The listing builds one solid part. Answer for the finished solid, in the listing's coordinates (mm). A direction names the side the tool comes from. Round coordinates to 2 decimals unless told otherwise and drop trailing zeros. Loops run counter-clockwise (first coordinate to the right, second up) from the corner with the lowest first, then second, coordinate; pieces in that order, holes last. Notation, with made-up numbers: (10.5, 72) -> (48.5, 72) arc R21 cw to (48.5, 110) -> close; hole circle Ø11 at (46, 27). An arc over 180 degrees is marked (long way). Write each question's results on one line, items separated by ' | '. Start each with the question number.
(1) Determine the mould class of faces 3 (the face through (-78.5, 508, -41)), 4 (the face through (-80, 508, -39)), 5 (the face through (-39, 508, -78.5)), 6 (the face through (-22, 1030.856, -1)) for opening direction X: released by +X, released by -X, zero draft, split by the parting line, or undercut.
(2) The part is cut by section A-A (z = -64.5). Determine the outline of the cut face in (x, y), plus the area to 3 significant figures.
(3) The part is cut by section C-C (y = 241.5). Determine the outline of the cut face in (x, z), plus the area to 3 significant figures.
(4) For faces 1 (the face through (-41, 508, -1.5)), 2 (the face through (-39, 508, 0)), determine the directions among +Z, -Z, +X, -X, +Y, -Y from which every point of the face is accessible in a straight line to the end or side of a thin tool.
(5) A straight line is drawn through the part: probe 1 along X at (y, z) = (925.5, -33.5). Find the intervals that lie inside material, in ascending order.
(6) The part is cut by section B-B (x = -15.5). Determine the outline of the cut face in (y, z).
Autodesk Inventor part; units mm, degrees
ref_plane "YZ Plane" through (0, 0, 0) normal (1, 0, 0) x (0, 1, 0)
ref_plane "XZ Plane" through (0, 0, 0) normal (0, 1, 0) x (-1, 0, 0)
ref_plane "XY Plane" through (0, 0, 0) normal (0, 0, 1) x (1, 0, 0)
sketch "Boceto1" plane through (0, 0, 0) normal (0, 1, 0) x (-1, 0, 0)
  line L0 (0, 0) -> (80, 0)
  line L1 (80, 0) -> (80, -80)
  line L2 (80, -80) -> (0, -80)
  line L3 (0, -80) -> (0, 0)
  line L4 (1.5, -78.5) -> (78.5, -78.5)
  line L5 (78.5, -78.5) -> (78.5, -1.5)
  line L6 (78.5, -1.5) -> (1.5, -1.5)
  line L7 (1.5, -1.5) -> (1.5, -78.5)
  line L8 (1.5, -78.5) -> (78.5, -1.5) construction
  line L9 (78.5, -78.5) -> (1.5, -1.5) construction
  point P0 (40, -40)
  dimension "d0" = 80
  dimension "d1" = 80
  dimension "d2" = 77
  dimension "d3" = 77
extrude "Extrusión1" add sketch "Boceto1" along normal blind 1030.856
properties part number "Pata_mesa"
Checked values:
1) face 3: undercut | face 4: released by -X | face 5: undercut | face 6: zero draft
2) outline: (-80, 0) -> (-78.5, 0) -> (-78.5, 1030.86) -> (-80, 1030.86) -> close; (-1.5, 0) -> (0, 0) -> (0, 1030.86) -> (-1.5, 1030.86) -> close | area: 3,090 mm2
3) outline: (-80, -80) -> (0, -80) -> (0, 0) -> (-80, 0) -> close; hole (-78.5, -78.5) -> (-1.5, -78.5) -> (-1.5, -1.5) -> (-78.5, -1.5) -> close | area: 471 mm2
4) face 1: +Y, -Y | face 2: +Z, +X, -X, +Y, -Y
5) probe 1: x = -80 to -78.5, -1.5 to 0
6) outline: (0, -80) -> (1030.86, -80) -> (1030.86, -78.5) -> (0, -78.5) -> close; (0, -1.5) -> (1030.86, -1.5) -> (1030.86, 0) -> (0, 0) -> close
